Can you work these out from the model? Positions are in its coordinate system, mm. A direction names the side the tool comes from. Give positions to 0.01 mm unless a question says otherwise; leave off trailing zeros. Write each loop counter-clockwise with the first axis right and the second up, starting at its lowest first coordinate (ties: lowest second). Pieces come first, ordered by that corner, then holes.
from build123d import *

# Parameters (mm, degrees)
FILLET1_R    = 1
SKETCH3_W    = 1.03
SKETCH3_H    = 4.4
SKETCH4_W    = 1.03
SKETCH4_H    = 1.897120746
RECPAT_COUNT = 2
RECPAT_ANGLE = 90


with BuildPart() as part:
    # BodySke → Base-Revolve (revolve)
    with BuildSketch(Plane.XY):
        Polygon((0, 0), (0, 4.2), (0.5, 4.2), (2.7, 2), (8, 2), (8, 0), align=None)
    revolve(axis=Axis((-6.35, 0, 0), (1, 0, 0)))

    # Fillet1
    fillet1_edges = [part.edges().sort_by_distance(p)[0] for p in [
        (2.7, -2, 0),
    ]]
    fillet(fillet1_edges, radius=FILLET1_R)

    # Sketch3 → Recess section 0
    with BuildSketch(Plane.ZY):
        Rectangle(SKETCH3_W, SKETCH3_H)
    # Sketch4 → Recess section 1
    with BuildSketch(Plane.ZY.offset(-2.51)):
        Rectangle(SKETCH4_W, SKETCH4_H)
    recess = loft(mode=Mode.SUBTRACT)

    # RecPat: Recess ×2 about axis
    recpat_axis = Axis((0, 0, 0), (1, 0, 0))
    for i in range(1, RECPAT_COUNT):
        add(recess.rotate(recpat_axis, i * RECPAT_ANGLE / (RECPAT_COUNT - 1)), mode=Mode.SUBTRACT)

    # RecCorSke → RecessCore (revolve, cut)
    with BuildSketch(Plane.XY):
        Polygon((0, 0), (0, 1.026516298), (2.51, 0.851), (2.786506661, 0), align=None)
    revolve(axis=Axis((-3.175, 0, 0), (1, 0, 0)), mode=Mode.SUBTRACT)


solid = part.part
(1) Imagine slicing it at A-A, the plane x = 7.25. Write out the boundary of the cut face in (y, z), plus the area to 3 significant figures.
Returned:
outline: circle Ø4 at (0, 0)
area: 12.6 mm2
(2) For faces 1 (the face through (1.273, 0.007, -1.566)), 2 (the face through (5.591, 1.847, -0.766)), 3 (the face through (8, 0, 0)), which set-ups out of +Z, -Z, +X, -X, +Y, -Y let a thin tool reach every point of the face, with its end or its side?
Returned:
face 1: -X
face 2: +X
face 3: +Z, -Z, +X, +Y, -Y
(3) If I drill on L1, parallel to Y at x = 6.5, z = 0; L2, parallel to X at y = 2.75, z = -1; L3, parallel to X at y = 2.75, z = 0, over which ranges is the centre line in solid material (lowest first)?
Returned:
L1: y = -2 to 2
L2: x = 0 to 1.77
L3: x = 0 to 1.95
(4) Will these pins go through, and if not, where does the flat tip stop? P1, Ø1, axis at x = 2, y = 0.5, coming from the -Z side; P2, Ø4, axis at x = 3.5, z = 3.5, coming from the +Y side; P3, Ø1.5, axis at x = 5, z = 0, coming from the +Y side.
Returned:
P1: stops at z = -3.17
P2: stops at y = 1.6
P3: stops at y = 2
(5) If we mould it in two halves opening along Z, with no side actions, what happens to faces 4 (the face through (0, -1, -1)), 5 (the face through (1.273, 1.566, 0.007)), 6 (the face through (0.254, 4.006, 1.262))? For each: +Z half, -Z half, draft (parallel to the pull), parting line (faces both ways), or undercut.
Returned:
face 4: draft
face 5: undercut
face 6: parting line
